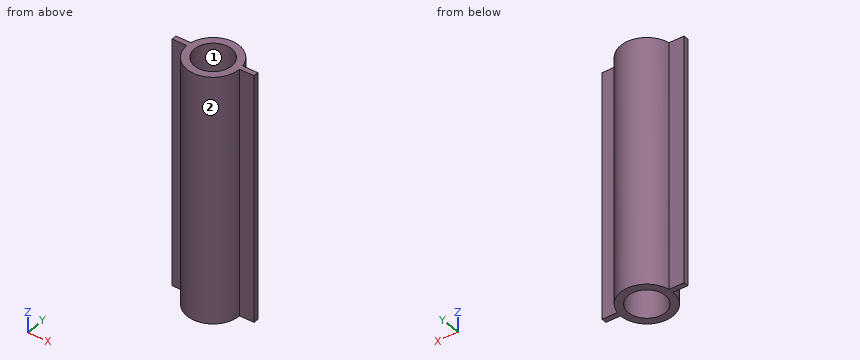
```python
from build123d import *

# Parameters (mm, degrees)
SKETCH2_R           = 3.75
BOSS_EXTRUDE1_DEPTH = 50


with BuildPart() as part:
    # Sketch2 → Boss-Extrude1 (new body)
    with BuildSketch(Plane.XY):
        with BuildLine():
            Line((-8.153882032, 0), (-5.25, 0))
            ThreePointArc((-5.25, 0), (0, -5.25), (5.25, 0))
            Line((5.25, 0), (8.153882032, 0))
            Line((8.153882032, 0), (8.153882032, 1))
            Line((8.153882032, 1), (5.153882032, 1))
            ThreePointArc((5.153882032, 1), (0, 5.25), (-5.153882032, 1))
            Line((-5.153882032, 1), (-8.153882032, 1))
            Line((-8.153882032, 1), (-8.153882032, 0))
        make_face()
        Circle(SKETCH2_R, mode=Mode.SUBTRACT)
    extrude(amount=BOSS_EXTRUDE1_DEPTH)


solid = part.part
```
Check sheet for the modelled part. Datum: model origin and axes. Units: mm. Face numbers are marked on the shaded views. Round coordinates to 2 decimals unless told otherwise and drop trailing zeros. Loops run counter-clockwise (first coordinate to the right, second up) from the corner with the lowest first, then second, coordinate; pieces in that order, holes last. Notation, with made-up numbers: (-13.5, 37) -> (-5.5, 37) arc R23 cw to (-5.5, 50) -> close; hole circle Ø8 at (-1, 83.5). An arc over 180 degrees is marked (long way). Answer in a Markdown table with one row per item.
Q1. Release check for a two-part mould opening along X. For the marked faces 1 and 2 record: released by +X, released by -X, zero draft, split by the parting line, or undercut.
Data:
| item | result |
|---|---|
| face 1 | undercut |
| face 2 | split by the parting line |
Q2. Thickness scan on L1, parallel to Y at x = -6.25, z = 32; L2, parallel to X at y = 1.75, z = 30.5; L3, parallel to X at y = -1, z = 28.5. Record the ranges inside material, lowest first.
Data:
| item | result |
|---|---|
| L1 | y = 0 to 1 |
| L2 | x = -4.95 to -3.32, 3.32 to 4.95 |
| L3 | x = -5.15 to -3.61, 3.61 to 5.15 |
Q3. Sectioned sample at C-C on z = 46. Enter the section's corners in (x, y), then the cut area to 3 significant figures.
Data:
| item | result |
|---|---|
| outline | (-8.15, 0) -> (-5.25, 0) arc R5.25 ccw to (5.25, 0) -> (8.15, 0) -> (8.15, 1) -> (5.15, 1) arc R5.25 ccw to (-5.15, 1) -> (-8.15, 1) -> close; hole circle Ø7.5 at (0, 0) |
| area | 48.3 mm^2 |
Q4. Go/stop test with flat-tipped pins: P1, Ø3.5, axis at x = -6.5, z = 20, coming from the +Y side; P2, Ø4.5, axis at x = 0, y = 0, coming from the +Z side; P3, Ø2, axis at x = 2, z = 33.5, coming from the +Y side; P4, Ø1.5, axis at x = 4.5, z = 20.5, coming from the +Y side. Record where each tip stops, or that it passes through.
Data:
| item | result |
|---|---|
| P1 | stops at y = 2.24 |
| P2 | passes through |
| P3 | stops at y = 5.15 |
| P4 | stops at y = 3.67 |
Q5. Sectioned sample at D-D on x = -6. Enter the section's corners in (y, z), then the cut area to 3 significant figures.
Data:
| item | result |
|---|---|
| outline | (0, 0) -> (1, 0) -> (1, 50) -> (0, 50) -> close |
| area | 50.0 mm^2 |
Q6. Sectioned sample at B-B on y = -0.75. Enter the section's corners in (x, z).
Data:
| item | result |
|---|---|
| outline | (-5.2, 0) -> (-3.67, 0) -> (-3.67, 50) -> (-5.2, 50) -> close; (3.67, 0) -> (5.2, 0) -> (5.2, 50) -> (3.67, 50) -> close |
Q7. Sectioned sample at A-A on x = 0. Enter the section's corners in (y, z), then the cut area to 3 significant figures.
Data:
| item | result |
|---|---|
| outline | (-5.25, 0) -> (-3.75, 0) -> (-3.75, 50) -> (-5.25, 50) -> close; (3.75, 0) -> (5.25, 0) -> (5.25, 50) -> (3.75, 50) -> close |
| area | 150 mm^2 |
